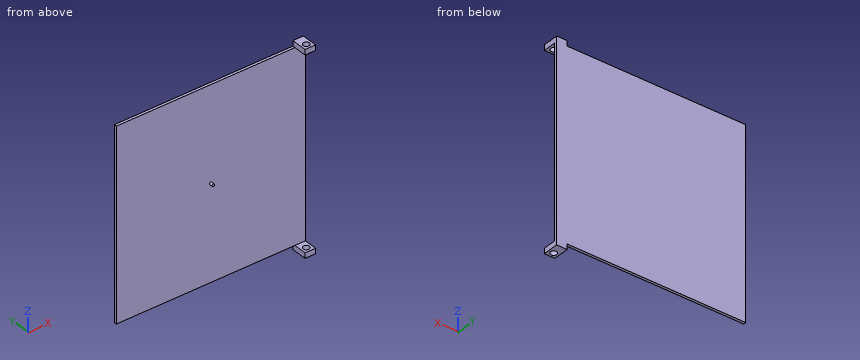
from build123d import *

# Parameters (mm, degrees)
SKETCH1_W           = 457.2
SKETCH1_H           = 228.6
BOSS_EXTRUDE1_DEPTH = 6.35
SKETCH2_W           = 25.4
SKETCH2_H           = 38.1
SKETCH2_R           = 7.62
BOSS_EXTRUDE2_DEPTH = 12.7
SKETCH4_R           = 3.175
BOSS_EXTRUDE4_DEPTH = 7.62


with BuildPart() as part:
    # Sketch1 → Boss-Extrude1 (new body)
    with BuildSketch(Plane(origin=(0, 0, 0), x_dir=(1, 0, 0), z_dir=(0, 1, 0))):
        with Locations((228.6, 114.3)):
            Rectangle(SKETCH1_W, SKETCH1_H)
    boss_extrude1 = extrude(amount=BOSS_EXTRUDE1_DEPTH)

    # Sketch2 → Boss-Extrude2 (add)
    with BuildSketch(Plane.XY):
        with Locations((444.5, -12.7)):
            Rectangle(SKETCH2_W, SKETCH2_H)
        with Locations((444.5, -19.05)):
            Circle(SKETCH2_R, mode=Mode.SUBTRACT)
    boss_extrude2 = extrude(amount=BOSS_EXTRUDE2_DEPTH)

    # Mirror3: Boss-Extrude1, Boss-Extrude2 across plane
    add(boss_extrude1.mirror(Plane(origin=(0, 6.35, -228.6), x_dir=(1, 0, 0), z_dir=(0, 0, 1))))
    add(boss_extrude2.mirror(Plane(origin=(0, 6.35, -228.6), x_dir=(1, 0, 0), z_dir=(0, 0, 1))))

    # Sketch4 → Boss-Extrude4 (add)
    with BuildSketch(Plane.XZ):
        with Locations((228.6, -228.6)):
            Circle(SKETCH4_R)
    extrude(amount=BOSS_EXTRUDE4_DEPTH)


solid = part.part
Can you work these out from the model? Positions are in its coordinate system, mm. Round coordinates to 2 decimals unless told otherwise and drop trailing zeros. Loops run counter-clockwise (first coordinate to the right, second up) from the corner with the lowest first, then second, coordinate; pieces in that order, holes last. Notation, with made-up numbers: (83.5, 37) - (116.5, 37) arc R28 cw to (116.5, 66) - close; hole circle Ø1 at (33, 39). An arc over 180 degrees is marked (long way). Answer in a Markdown table with one row per item. Add a question column.
Q1. I need wall thicknesses on L1, parallel to Y at x = 444.5, z = -463.75; L2, parallel to Y at x = 196, z = -443; L3, parallel to Z at x = 200.5, y = 1. Which ranges of each line are inside material? Lowest first, please.
Q2. I want a section at A-A on x = 444.5. List the corners of the cut face in (y, z) for me, and give its area (3 significant figures).
Q3. I want a section at B-B on z = -336. List the corners of the cut face in (x, y) for me, and give its area (3 significant figures).
Q4. For pin 1 Ø5 at (x, y) = (205, 4) entering from -Z; pin 2 Ø7 at (x, y) = (281, 3.5) entering from +Z; pin 3 Ø10 at (y, z) = (-21, -462.5) entering from -X, each with a flat end and sliding along its axis, tell me the tip position at first contact or that it passes through.
Q5. I want a section at C-C on x = 212.5. List the corners of the cut face in (y, z) for me, and give its area (3 significant figures).
A:
| question | item | result |
|---|---|---|
| 1 | L1 | -31.75 to -26.67, -11.43 to 6.35 |
| 1 | L2 | 0 to 6.35 |
| 1 | L3 | -457.2 to 0 |
| 2 | outline | (-31.75, -469.9) - (-26.67, -469.9) - (-26.67, -457.2) - (-31.75, -457.2) - close; (-31.75, 0) - (-26.67, 0) - (-26.67, 12.7) - (-31.75, 12.7) - close; (-11.43, -469.9) - (6.35, -469.9) - (6.35, 12.7) - (-11.43, 12.7) - (-11.43, 0) - (0, 0) - (0, -457.2) - (-11.43, -457.2) - close |
| 2 | area | 3,480 mm^2 |
| 3 | outline | (0, 0) - (457.2, 0) - (457.2, 6.35) - (0, 6.35) - close |
| 3 | area | 2,900 mm^2 |
| 4 | pin 1 | z = -457.2 |
| 4 | pin 2 | z = 0 |
| 4 | pin 3 | x = 431.8 |
| 5 | outline | (0, -457.2) - (6.35, -457.2) - (6.35, 0) - (0, 0) - close |
| 5 | area | 2,900 mm^2 |
